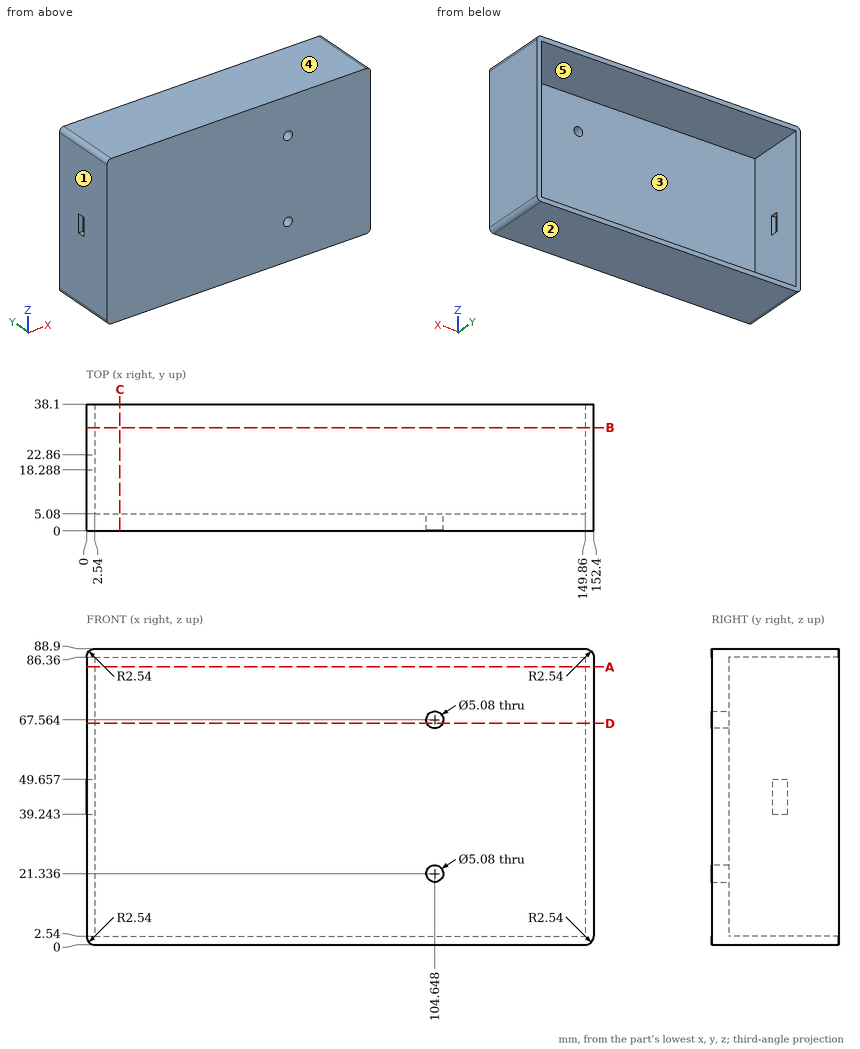
Could you check a few things on this drawing? It's one solid part, dimensions in mm from its lowest x, y, z. A direction names the side the tool comes from. Coordinates: 2 decimals unless noted, no trailing zeros. Order: outer loops, then holes, each group sorted by start corner. A loop starts at its lowest first (then second) coordinate and runs counter-clockwise, first axis right, second up. Notation, with made-up numbers: M 74.25,3.25 L 119.25,3.25 A11 ccw 119.25,24.25 Z; hole C 81,22 d8. An arc over 180 degrees is marked long. Use one line per item in the form item = value. Start each with the question number.
1. We'd pull the mould along X, two halves only. Please class the marked faces 1, 2 and 3: +X half, -X half, draft (parallel to the pull), parting line (faces both ways), or undercut.
2. Suppose I cut it at A-A on z = 83.5. Write out the boundary of the cut face in (x, y), then the cut area to 3 significant figures.
3. For pin 1 (1.5 mm diameter, centred on x = 65.5, z = 57.5, fed in from +Y); pin 2 (2 mm diameter, centred on x = 0.5, y = 20.5, fed in from +Z), each with a flat end and sliding along its axis, tell me the tip position at first contact or that it passes through.
4. Suppose I cut it at C-C on x = 10. Write out the boundary of the cut face in (y, z), then the cut area to 3 significant figures.
5. On a 3-axis mill with a long thin cutter (end or side, diameter ignored), from which of +Z, -Z, +X, -X, +Y, -Y can I reach the whole of each face in a straight line? I mean the marked faces 4 and 5. Say none if no direction works.
6. Suppose I cut it at B-B on y = 31. Write out the boundary of the cut face in (x, z).
7. Suppose I cut it at D-D on z = 66.5. Write out the boundary of the cut face in (x, y).
8. Please list where these lines run through material, in increasing order: line 1 (X direction, y = 18, z = 38); line 2 (Z direction, x = 142.5, y = 35.5); line 3 (Y direction, x = 84, z = 43).
Geometry says:
q1.face_1 = -X half
q1.face_2 = draft
q1.face_3 = undercut
q2.outline = M 0,0 L 152.4,0 L 152.4,38.1 L 149.86,38.1 L 149.86,5.08 L 2.54,5.08 L 2.54,38.1 L 0,38.1 Z
q2.area = 942 mm^2
q3.pin_1 = 5.08
q3.pin_2 = 88.68
q4.outline = M 0,0 L 38.1,0 L 38.1,2.54 L 5.08,2.54 L 5.08,86.36 L 38.1,86.36 L 38.1,88.9 L 0,88.9 Z
q4.area = 619 mm^2
q5.face_4 = +Z, +X, -X, +Y, -Y
q5.face_5 = +Y
q6.outline = M 0,2.54 A2.54 ccw 2.54,0 L 149.86,0 A2.54 ccw 152.4,2.54 L 152.4,86.36 A2.54 ccw 149.86,88.9 L 2.54,88.9 A2.54 ccw 0,86.36 Z; hole M 2.54,2.54 L 149.86,2.54 L 149.86,86.36 L 2.54,86.36 Z
q7.outline = M 0,0 L 102.34,0 L 102.34,5.08 L 2.54,5.08 L 2.54,38.1 L 0,38.1 Z; M 106.95,0 L 152.4,0 L 152.4,38.1 L 149.86,38.1 L 149.86,5.08 L 106.95,5.08 Z
q8.line_1 = 0 to 2.54, 149.86 to 152.4
q8.line_2 = 0 to 2.54, 86.36 to 88.9
q8.line_3 = 0 to 5.08
